Geometry check sheet. Reference: the model listing, model coordinates, mm. A direction names the side the tool comes from. Coordinates: 2 decimals unless noted, no trailing zeros. Order: outer loops, then holes, each group sorted by start corner. A loop starts at its lowest first (then second) coordinate and runs counter-clockwise, first axis right, second up. Notation, with made-up numbers: (78, -19.75) - (113, -19.75) arc R25 ccw to (113, 14.25) - close; hole circle Ø5 at (49, 17.5). An arc over 180 degrees is marked (long way). One line per item, written item: value. Start each with the question number.
```python
from build123d import *

# Parameters (mm, degrees)
HOLE_WIZARD_M6_1_D     = 5
HOLE_WIZARD_M6_1_DEPTH = 17
HOLE_WIZARD_M6_1_TIP   = 1.502151548
CUT_EXTRUDE_1_DEPTH    = 10
CUT_EXTRUDE_2_DEPTH    = 10
CHAMFER_1_SIZE         = 1


with BuildPart() as part:
    # 草图1 → 旋转1 (revolve)
    with BuildSketch(Plane.XY, mode=Mode.PRIVATE) as revolve_1_sk:
        Polygon((0, 0), (0, 17.5), (45, 17.5), (75, 17.5), (75, 25), (105, 25), (105, 22.5), (140, 22.5), (140, 21), (170, 21), (170, 20), (235, 20), (235, 17.5), (253, 17.5), (253, 0), align=None)
    revolve(revolve_1_sk.sketch.rotate(Axis((0, 0, 0), (1, 0, 0)), 90), axis=Axis((0, 0, 0), (1, 0, 0)))

    # M6 螺纹孔1
    with Locations(Plane(origin=(0, 0, 0), x_dir=(0, 0, -1), z_dir=(-1, 0, 0))):
        with Locations((0, 0)):
            Hole(HOLE_WIZARD_M6_1_D / 2, depth=HOLE_WIZARD_M6_1_DEPTH)
            with Locations((0, 0, -(HOLE_WIZARD_M6_1_DEPTH + HOLE_WIZARD_M6_1_TIP / 2))):  # 118° drill point
                Cone(0, HOLE_WIZARD_M6_1_D / 2, HOLE_WIZARD_M6_1_TIP, mode=Mode.SUBTRACT)

    # 草图4 → 切除-拉伸1 (cut)
    with BuildSketch(Plane.XY.offset(17)):
        with BuildLine():
            Line((113, 7), (132, 7))
            ThreePointArc((132, 7), (139, 0), (132, -7))
            Line((132, -7), (113, -7))
            ThreePointArc((113, -7), (106, 0), (113, 7))
        make_face()
    extrude(amount=CUT_EXTRUDE_1_DEPTH, mode=Mode.SUBTRACT)

    # 草图5 → 切除-拉伸2 (cut)
    with BuildSketch(Plane.XY.offset(12.5)):
        with BuildLine():
            Line((8, 5), (38, 5))
            ThreePointArc((38, 5), (43, 0), (38, -5))
            Line((38, -5), (8, -5))
            ThreePointArc((8, -5), (3, 0), (8, 5))
        make_face()
    extrude(amount=CUT_EXTRUDE_2_DEPTH, mode=Mode.SUBTRACT)

    # 倒角1
    chamfer_1_edges = [part.edges().sort_by_distance(p)[0] for p in [
        (253, 0, -17.5),
        (0, 0, -17.5),
    ]]
    chamfer(chamfer_1_edges, length=CHAMFER_1_SIZE)


solid = part.part
```
Q1. Cross-section at A-A, the plane x = 60.5. Enter the section's corners in (y, z).
Q2. Material ranges on probe 1 along Y at (x, z) = (7.5, 0); probe 2 along X at (y, z) = (-22.5, 7.5); probe 3 along X at (y, z) = (-20, -2.5), recorded low to high.
Q3. Cross-section at B-B, the plane x = 144. Enter the section's corners in (y, z), and give its area (3 significant figures).
Q4. Set-up check for faces 5 (the flat face through (105, -3.82, -22.34)), 6 (the flat face through (75, 5, 17)), 7 (the flat face through (23, 5, 15)): record each of +Z, -Z, +X, -X, +Y, -Y from which the full face is reachable in a straight line by a thin tool's end or side.
Q5. Release check for a two-part mould opening along X. For faces 1 (the flat face through (170, 8, 19)), 2 (the flat face through (123, 0, 17)), 3 (the cylindrical face through (8.62, 2.44, -0.54)), 4 (the flat face through (122, 7, 19)) record: released by +X, released by -X, zero draft, split by the parting line, or undercut.
Q6. Gauge pin test, flat ends, axial feed: P1, Ø1.5, axis at x = 110.5, z = 7, coming from the -Y side; P2, Ø3.5, axis at x = 28, z = 14, coming from the -Y side; P3, Ø10, axis at x = 189, z = 0.5, coming from the +Y side. Record the tip position at first contact, or that the pin passes through.
Check result:
1. outline: circle Ø35 at (0, 0)
2. probe 1: y = -17.5 to -2.5, 2.5 to 17.5
2. probe 2: x = 75 to 105
2. probe 3: x = 75 to 170
3. outline: circle Ø42 at (0, 0)
3. area: 1,390 mm2
4. face 5: +X
4. face 6: -X
4. face 7: +Z
5. face 1: released by +X
5. face 2: undercut
5. face 3: zero draft
5. face 4: undercut
6. P1: stops at y = -21.61
6. P2: stops at y = -12.5
6. P3: stops at y = 20
